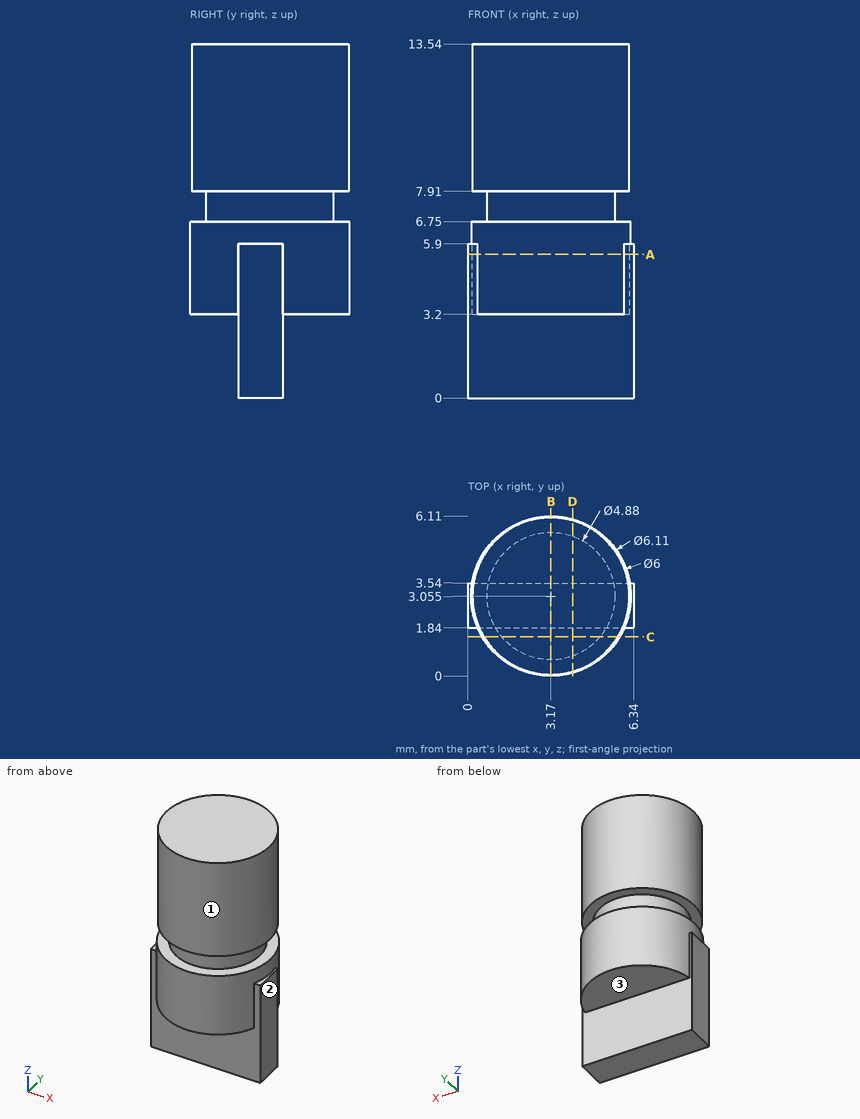
Study the drawing (mm; zero at the part's minimum x, y, z) and answer. A direction names the side the tool comes from. Coordinates: 2 decimals unless noted, no trailing zeros. Loops run counter-clockwise (first coordinate to the right, second up) from the corner with the lowest first, then second, coordinate; pieces in that order, holes last. Notation, with made-up numbers: M -27.5,4 L -12.5,4 A18 cw -12.5,30 Z; hole C 46.25,10 d2. An arc over 180 degrees is marked long. Answer in a Markdown table with one row per item. Add a question column.
1. Find section D-D, the plane x = 4. Write down the section's boundary in (y, z).
2. Flat-ended cylindrical pins translate along their axes: P1, Ø2, axis at x = 3, y = 0.5, coming from the -Z side; P2, Ø1.8, axis at x = 4.5, y = 4, coming from the -Z side; P3, Ø3, axis at y = 3.5, z = 7.5, coming from the -X side (3 decimals); P4, Ø1.8, axis at x = 4.5, z = 2, coming from the -Y side. Find the tip coordinate at first contact, or state that the pin passes through.
3. Find section B-B, the plane x = 3.17. Write down the section's boundary in (y, z) (3 decimals).
4. Find section C-C, the plane y = 1.5. Write down the section's boundary in (x, z), then the cut area to 3 significant figures.
5. Find section A-A, the plane z = 5.5. Write down the section's boundary in (x, y) (3 decimals), then the cut area to 3 significant figures.
6. A tool of negligible diameter and unlimited length cuts with its end or side. For the marked faces 1, 2 and 3, from which of +Z, -Z, +X, -X, +Y, -Y can it reach the whole face along a straight path? Write none if from no direction.
7. Consider L1, parallel to Z at x = 5.75, y = 2.5; L2, parallel to Z at x = 5.75, y = 4; L3, parallel to Y at x = 3.75, z = 3.75. Determine where each line is inside the solid, lowest interval first.
Reported:
| question | item | result |
|---|---|---|
| 1 | outline | M 0.11,3.2 L 1.84,3.2 L 1.84,0 L 3.54,0 L 3.54,3.2 L 6,3.2 L 6,6.75 L 5.35,6.75 L 5.35,7.91 L 5.94,7.91 L 5.94,13.54 L 0.17,13.54 L 0.17,7.91 L 0.76,7.91 L 0.76,6.75 L 0.11,6.75 Z |
| 2 | P1 | stops at z = 3.2 |
| 2 | P2 | stops at z = 0 |
| 2 | P3 | stops at x = 0.115 |
| 2 | P4 | stops at y = 1.84 |
| 3 | outline | M 0,3.2 L 1.84,3.2 L 1.84,0 L 3.54,0 L 3.54,3.2 L 6.11,3.2 L 6.11,6.75 L 5.495,6.75 L 5.495,7.91 L 6.055,7.91 L 6.055,13.54 L 0.055,13.54 L 0.055,7.91 L 0.615,7.91 L 0.615,6.75 L 0,6.75 Z |
| 4 | outline | M 0.54,3.2 L 5.8,3.2 L 5.8,6.75 L 5.05,6.75 L 5.05,7.91 L 5.74,7.91 L 5.74,13.54 L 0.6,13.54 L 0.6,7.91 L 1.29,7.91 L 1.29,6.75 L 0.54,6.75 Z |
| 4 | area | 51.9 mm^2 |
| 5 | outline | M 0,1.84 L 0.367,1.84 A3.055 ccw 5.973,1.84 L 6.34,1.84 L 6.34,3.54 L 6.186,3.54 A3.055 ccw 0.154,3.54 L 0,3.54 Z |
| 5 | area | 29.9 mm^2 |
| 6 | face 1 | +Z |
| 6 | face 2 | +Z, -Z, +X, +Y, -Y |
| 6 | face 3 | -Z, +X, -X, +Y |
| 7 | L1 | z = 0 to 6.75, 7.91 to 13.54 |
| 7 | L2 | z = 3.2 to 6.75, 7.91 to 13.54 |
| 7 | L3 | y = 0.06 to 6.05 |
